Build history of the part. All positions in model axes, mm. A direction names the side the tool comes from. Give positions to 0.01 mm unless a question says otherwise; leave off trailing zeros. Write each loop counter-clockwise with the first axis right and the second up, starting at its lowest first coordinate (ties: lowest second). Pieces come first, ordered by that corner, then holes. Notation, with made-up numbers: (83, 62.25) -> (124, 62.25) arc R23 cw to (124, 72.25) -> close; hole circle Ø6 at (13.25, -26.75). An arc over 180 degrees is marked (long way). Write item = value, one per line. Start each with the question number.
Q1. Wall check: line 1 (X direction, y = -4, z = 5.5); line 2 (X direction, y = 8, z = 3); line 3 (Y direction, x = 14.5, z = 5.5). Give the ranges that are in metal, low to high.
Q2. Saw through at D-D, the plane x = 12. List the corners of the cut face in (y, z).
Q3. Mould opens along Y. For faces 1 (the face through (33.43, 19.4, 3.3)), 2 (the face through (3, -2, 3)), 3 (the face through (28.146, 7.426, 3.296)) say: pulls with the +Y half, pulls with the -Y half, needs draft (parallel to the pull), parting line crosses it, or undercut.
Q4. Drop flat-ended pins along their axis: P1, Ø1.3, axis at y = -2, z = 4, coming from the +X side; P2, Ø3.5, axis at x = 1.5, z = 3, coming from the +Y side; P3, Ø2.5, axis at x = 36, z = 1.5, coming from the -Y side. Give the stop position or say it passes through.
Q5. Saw through at B-B, the plane y = 6.75. List the corners of the cut face in (x, z), then the cut area to 3 significant figures.
Q6. Tool access for faces 4 (the face through (19, 13.5, 3)), 5 (the face through (34, -2, 3)), 6 (the face through (2, 13.5, 3)), 7 (the face through (30, 20, 3)), 8 (the face through (18, 0, 3)): list every direction of +Z, -Z, +X, -X, +Y, -Y with a clear straight run to the whole face (end or side of a thin tool).
Q7. Saw through at C-C, the plane z = 3.5. Give the number of separate pieces and of enclosed holes in the cut face, then the cut area to 3 significant figures.
Q8. Saw through at A-A, the plane y = -1.5. List the corners of the cut face in (x, z), then the cut area to 3 significant figures.
Autodesk Inventor part; units mm, degrees
ref_plane "YZ Plane" through (0, 0, 0) normal (1, 0, 0) x (0, 1, 0)
ref_plane "XZ Plane" through (0, 0, 0) normal (0, 1, 0) x (-1, 0, 0)
ref_plane "XY Plane" through (0, 0, 0) normal (0, 0, 1) x (1, 0, 0)
sketch "Sketch1" plane through (0, 0, 0) normal (0, 0, 1) x (1, 0, 0)
  line L0 (0, 0) -> (37, 0)
  line L1 (37, 0) -> (37, 13.5)
  line L2 (37, 13.5) -> (0, 13.5)
  line L3 (0, 13.5) -> (0, 0)
  dimension "d0" = 13.5
  dimension "d1" = 37
extrude "Extrusion1" add sketch "Sketch1" along normal blind 6.5
sketch "Sketch2" plane through (0, 0, 6.5) normal (0, 0, 1) x (1, 0, 0)
  line L0 (0, 0) -> (37, 0)
  line L1 (37, 13.5) -> (0, 13.5)
  line L2 (3, 13.5) -> (11, 13.5)
  line L3 (11, 13.5) -> (11, 18)
  line L4 (9, 20) -> (5, 20)
  line L5 (3, 18) -> (3, 13.5)
  line L6 (26, 13.5) -> (34, 13.5)
  line L7 (34, 13.5) -> (34, 18)
  line L8 (32, 20) -> (28, 20)
  line L9 (26, 18) -> (26, 13.5)
  line L10 (3, 0) -> (11, 0)
  line L11 (11, 0) -> (11, -4.5)
  line L12 (9, -6.5) -> (5, -6.5)
  line L13 (3, -4.5) -> (3, 0)
  line L14 (26, 0) -> (34, 0)
  line L15 (34, 0) -> (34, -4.5)
  line L16 (32, -6.5) -> (28, -6.5)
  line L17 (26, -4.5) -> (26, 0)
  arc A0 (5, 20) -> (3, 18) centre (5, 18) ccw
  arc A1 (11, 18) -> (9, 20) centre (9, 18) ccw
  arc A2 (28, 20) -> (26, 18) centre (28, 18) ccw
  arc A3 (34, 18) -> (32, 20) centre (32, 18) ccw
  arc A4 (3, -4.5) -> (5, -6.5) centre (5, -4.5) ccw
  arc A5 (9, -6.5) -> (11, -4.5) centre (9, -4.5) ccw
  arc A6 (26, -4.5) -> (28, -6.5) centre (28, -4.5) ccw
  arc A7 (32, -6.5) -> (34, -4.5) centre (32, -4.5) ccw
  line L18 (11, 15.75) -> (26, 15.75) construction
  point P0 (18.5, 15.75)
  point P1 (18.5, 13.5)
  dimension "d4" = 2
  dimension "d5" = 8
  dimension "d6" = 8
  dimension "d7" = 15
  dimension "d8" = 6.5
  dimension "d9" = 6.5
extrude "Extrusion2" add sketch "Sketch2" against normal blind 6.5
sketch "Sketch3" plane through (0, 0, 6.5) normal (0, 0, 1) x (1, 0, 0)
  line L0 (26, 13.5) -> (11, 13.5)
  line L1 (0, 13.5) -> (0, 0)
  line L2 (11, 6.75) -> (26, 6.75) construction
  circle A0 centre (11, 6.75) radius 2.25
  circle A1 centre (26, 6.75) radius 2.25
  point P0 (18.5, 6.75)
  point P1 (18.5, 13.5)
  point P2 (0, 6.75)
  dimension "d12" = 4.5
  dimension "d13" = 15
extrude "Extrusion3" cut sketch "Sketch3" against normal through all
equation "\"d9\" = d8"
properties part number "y_carriage_belt_iddler_holder" material "Plywood, Finish"
Report:
q1.line_1 = 3 to 11, 26 to 34
q1.line_2 = 0 to 9.13, 12.87 to 24.13, 27.87 to 37
q1.line_3 = 0 to 13.5
q2.outline = (0, 0) -> (4.73, 0) -> (4.73, 6.5) -> (0, 6.5) -> close; (8.77, 0) -> (13.5, 0) -> (13.5, 6.5) -> (8.77, 6.5) -> close
q3.face_1 = pulls with the +Y half
q3.face_2 = needs draft
q3.face_3 = undercut
q4.P1 = 34
q4.P2 = 18.97
q4.P3 = 0
q5.outline = (0, 0) -> (8.75, 0) -> (8.75, 6.5) -> (0, 6.5) -> close; (13.25, 0) -> (23.75, 0) -> (23.75, 6.5) -> (13.25, 6.5) -> close; (28.25, 0) -> (37, 0) -> (37, 6.5) -> (28.25, 6.5) -> close
q5.area = 182 mm2
q6.face_4 = +Z, -Z, +Y
q6.face_5 = +Z, -Z, +X, -Y
q6.face_6 = +Z, -Z, -X, +Y
q6.face_7 = +Z, -Z, +X, -X, +Y
q6.face_8 = +Z, -Z, -Y
q7.separate_pieces = 1
q7.enclosed_holes = 2
q7.area = 669 mm2
q8.outline = (3, 0) -> (11, 0) -> (11, 6.5) -> (3, 6.5) -> close; (26, 0) -> (34, 0) -> (34, 6.5) -> (26, 6.5) -> close
q8.area = 104 mm2
